Check sheet for the drawn part. Datum: minimum x, y, z corner. Units: mm. Coordinates: 2 decimals unless noted, no trailing zeros. Write each loop counter-clockwise with the first axis right and the second up, starting at its lowest first coordinate (ties: lowest second). Pieces come first, ordered by that corner, then holes. Notation, with made-up numbers: (-11, 84.25) -> (-5, 84.25) arc R31 ccw to (-5, 115.25) -> close; hole circle Ø2 at (80, 76.25). An arc over 180 degrees is marked (long way). Answer in a Markdown table with one row per item.
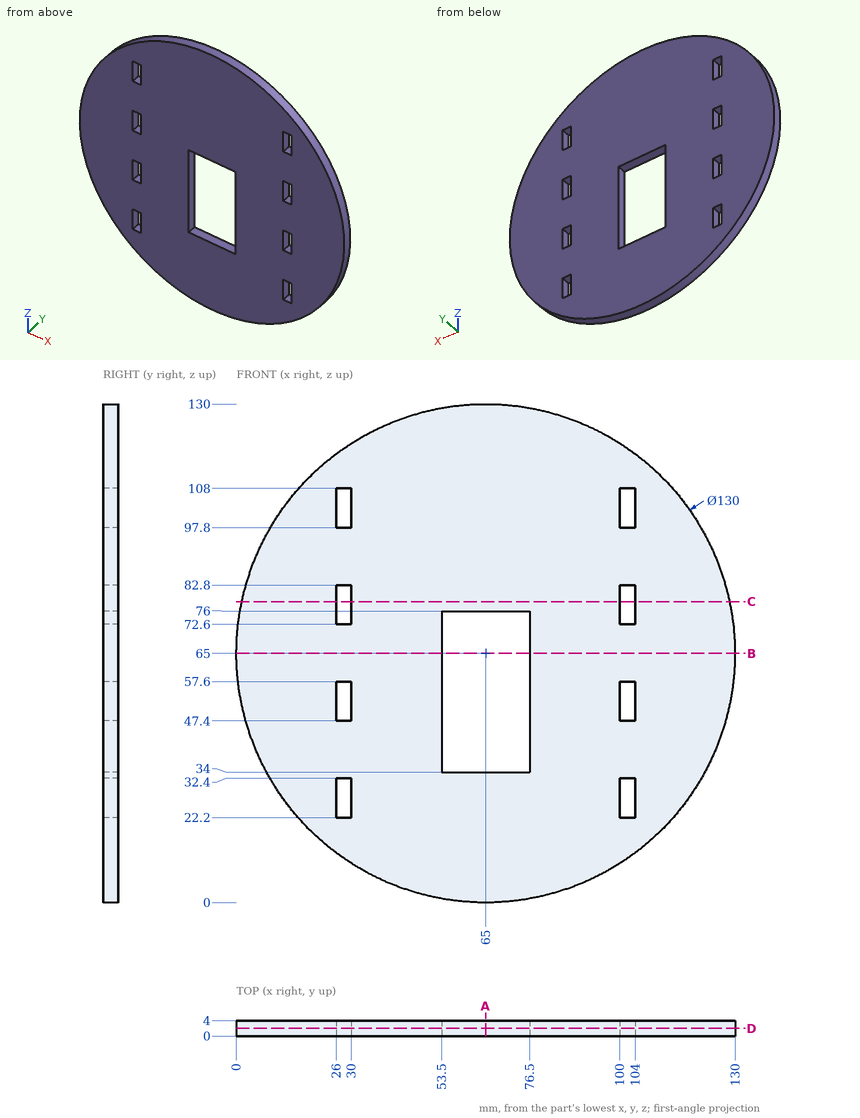
1. Sectioned sample at B-B, the plane z = 65. Record the cut outline in (x, y).
Findings below:
| item | result |
|---|---|
| outline | (0, 0) -> (53.5, 0) -> (53.5, 4) -> (0, 4) -> close; (76.5, 0) -> (130, 0) -> (130, 4) -> (76.5, 4) -> close |
2. Sectioned sample at A-A, the plane x = 65. Record the cut outline in (y, z), and give its area (3 significant figures).
Findings below:
| item | result |
|---|---|
| outline | (0, 0) -> (4, 0) -> (4, 34) -> (0, 34) -> close; (0, 76) -> (4, 76) -> (4, 130) -> (0, 130) -> close |
| area | 352 mm² |
3. Sectioned sample at D-D, the plane y = 2. Count the separate pieces of the cut face and the enclosed holes in it, and give its area (3 significant figures).
Findings below:
| item | result |
|---|---|
| separate pieces | 1 |
| enclosed holes | 9 |
| area | 12,000 mm² |
4. Material ranges on probe 1 along X at (y, z) = (2.55, 65.5); probe 2 along X at (y, z) = (1.35, 101.5); probe 3 along X at (y, z) = (2.8, 24), recorded low to high. Write a range as from..to.
Findings below:
| item | result |
|---|---|
| probe 1 | x = 0..53.5, 76.5..130 |
| probe 2 | x = 11.22..26, 30..100, 104..118.78 |
| probe 3 | x = 14.56..26, 30..100, 104..115.44 |
5. Sectioned sample at C-C, the plane z = 78.5. Record the cut outline in (x, y).
Findings below:
| item | result |
|---|---|
| outline | (1.42, 0) -> (26, 0) -> (26, 4) -> (1.42, 4) -> close; (30, 0) -> (100, 0) -> (100, 4) -> (30, 4) -> close; (104, 0) -> (128.58, 0) -> (128.58, 4) -> (104, 4) -> close |
6. Go/stop test with flat-tipped pins: pin 1 (2 mm diameter, centred on y = 2, z = 50.5, fed in from -X); pin 2 (2 mm diameter, centred on y = 2, z = 103.5, fed in from -X); pin 3 (1 mm diameter, centred on x = 67.5, y = 2, fed in from -Z). Record where each tip stops, or that it passes through.
Findings below:
| item | result |
|---|---|
| pin 1 | stops at x = 1.42 |
| pin 2 | stops at x = 11.91 |
| pin 3 | stops at z = 0.03 |
